Verification items for the finished model (mm, model axes). Give positions to 0.01 mm unless a question says otherwise; leave off trailing zeros. Loops run counter-clockwise (first coordinate to the right, second up) from the corner with the lowest first, then second, coordinate; pieces in that order, holes last. Notation, with made-up numbers: (14, 28) - (34, 28) arc R19 ccw to (34, 65) - close; hole circle Ø9 at (8, 21). An arc over 180 degrees is marked (long way). Answer in a Markdown table with one row per item.
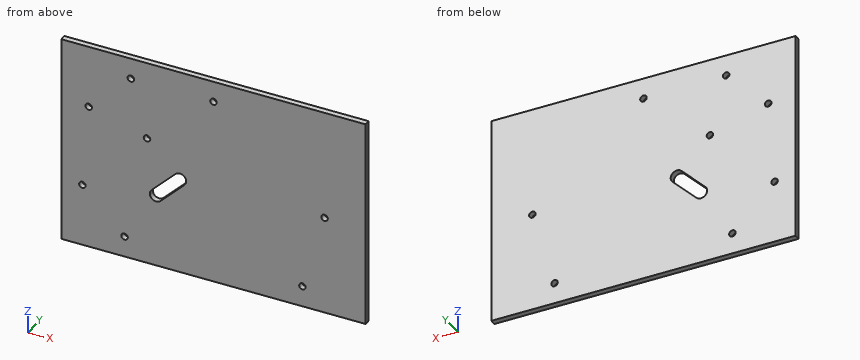
```python
from build123d import *

# Parameters (mm, degrees)
SKETCH1_W           = 144.5
SKETCH1_H           = 100
SKETCH1_R           = 1.55
BOSS_EXTRUDE1_DEPTH = 2.8
CUT_EXTRUDE1_REACH  = 4.8
CUT_EXTRUDE2_REACH  = 4.8
SKETCH3_R           = 1.55
CUT_EXTRUDE3_REACH  = 4.8
SKETCH4_R           = 1.55


with BuildPart() as part:
    # Sketch1 → Boss-Extrude1 (new body)
    with BuildSketch(Plane(origin=(0, 0, 0), x_dir=(1, 0, 0), z_dir=(0, 1, 0))):
        Rectangle(SKETCH1_W, SKETCH1_H)
        with Locations((-59.25, -20)):
            Circle(SKETCH1_R, mode=Mode.SUBTRACT)
        with Locations((-39.25, -40)):
            Circle(SKETCH1_R, mode=Mode.SUBTRACT)
        with Locations((-31.57233047, -12.32233047)):
            Circle(SKETCH1_R, mode=Mode.SUBTRACT)
    extrude(amount=BOSS_EXTRUDE1_DEPTH)

    # Sketch2 → Cut-Extrude1 (cut, up to next)
    with BuildSketch(Plane(origin=(0, 2.8, 0), x_dir=(1, 0, 0), z_dir=(0, 1, 0)), mode=Mode.PRIVATE) as cut_extrude1_sk1:
        with BuildLine():
            Line((-25.128679656, 17.121320344), (-13.814971157, 5.807611845))
            ThreePointArc((-13.814971157, 5.807611845), (-13.814971157, 1.564971157), (-18.057611845, 1.564971157))
            Line((-18.057611845, 1.564971157), (-29.371320344, 12.878679656))
            ThreePointArc((-29.371320344, 12.878679656), (-29.371320344, 17.121320344), (-25.128679656, 17.121320344))
        make_face()
    cut_extrude1_tool1 = extrude(cut_extrude1_sk1.sketch, amount=-CUT_EXTRUDE1_REACH, mode=Mode.PRIVATE) & part.part
    add(cut_extrude1_tool1.solids().sort_by_distance((-21.593146, 2.8, -9.343146))[0], mode=Mode.SUBTRACT)

    # Sketch3 → Cut-Extrude2 (cut, up to next)
    with BuildSketch(Plane(origin=(0, 2.8, 0), x_dir=(1, 0, 0), z_dir=(0, 1, 0)), mode=Mode.PRIVATE) as cut_extrude2_sk1:
        with Locations((-62.25, 20)):
            Circle(SKETCH3_R)
    cut_extrude2_tool1 = extrude(cut_extrude2_sk1.sketch, amount=-CUT_EXTRUDE2_REACH, mode=Mode.PRIVATE) & part.part
    add(cut_extrude2_tool1.solids().sort_by_distance((-62.25, 2.8, -20))[0], mode=Mode.SUBTRACT)
    # Sketch3 → Cut-Extrude2 (cut, up to next)
    with BuildSketch(Plane(origin=(0, 2.8, 0), x_dir=(1, 0, 0), z_dir=(0, 1, 0)), mode=Mode.PRIVATE) as cut_extrude2_sk2:
        with Locations((-42.25, 40)):
            Circle(SKETCH3_R)
    cut_extrude2_tool2 = extrude(cut_extrude2_sk2.sketch, amount=-CUT_EXTRUDE2_REACH, mode=Mode.PRIVATE) & part.part
    add(cut_extrude2_tool2.solids().sort_by_distance((-42.25, 2.8, -40))[0], mode=Mode.SUBTRACT)
    # Sketch3 → Cut-Extrude2 (cut, up to next)
    with BuildSketch(Plane(origin=(0, 2.8, 0), x_dir=(1, 0, 0), z_dir=(0, 1, 0)), mode=Mode.PRIVATE) as cut_extrude2_sk3:
        with Locations((42.25, 40)):
            Circle(SKETCH3_R)
    cut_extrude2_tool3 = extrude(cut_extrude2_sk3.sketch, amount=-CUT_EXTRUDE2_REACH, mode=Mode.PRIVATE) & part.part
    add(cut_extrude2_tool3.solids().sort_by_distance((42.25, 2.8, -40))[0], mode=Mode.SUBTRACT)
    # Sketch3 → Cut-Extrude2 (cut, up to next)
    with BuildSketch(Plane(origin=(0, 2.8, 0), x_dir=(1, 0, 0), z_dir=(0, 1, 0)), mode=Mode.PRIVATE) as cut_extrude2_sk4:
        with Locations((0, -40)):
            Circle(SKETCH3_R)
    cut_extrude2_tool4 = extrude(cut_extrude2_sk4.sketch, amount=-CUT_EXTRUDE2_REACH, mode=Mode.PRIVATE) & part.part
    add(cut_extrude2_tool4.solids().sort_by_distance((0, 2.8, 40))[0], mode=Mode.SUBTRACT)

    # Sketch4 → Cut-Extrude3 (cut, up to next)
    with BuildSketch(Plane(origin=(0, 2.8, 0), x_dir=(1, 0, 0), z_dir=(0, 1, 0)), mode=Mode.PRIVATE) as cut_extrude3_sk1:
        with Locations((52.75, 2.56)):
            Circle(SKETCH4_R)
    cut_extrude3_tool1 = extrude(cut_extrude3_sk1.sketch, amount=-CUT_EXTRUDE3_REACH, mode=Mode.PRIVATE) & part.part
    add(cut_extrude3_tool1.solids().sort_by_distance((52.75, 2.8, -2.56))[0], mode=Mode.SUBTRACT)


solid = part.part
```
Q1. Thickness scan on line 1 (X direction, y = 0.9, z = 40); line 2 (Z direction, x = -39.25, y = 0.85); line 3 (X direction, y = 1.45, z = -40). Record the ranges inside material, lowest first.
Completed:
| item | result |
|---|---|
| line 1 | -72.25 to -40.8, -37.7 to -1.55, 1.55 to 72.25 |
| line 2 | -50 to 38.45, 41.55 to 50 |
| line 3 | -72.25 to -43.8, -40.7 to 40.7, 43.8 to 72.25 |
Q2. Sectioned sample at B-B (z = 20). Record the cut outline in (x, y), and give its area (3 significant figures).
Completed:
| item | result |
|---|---|
| outline | (-72.25, 0) - (-60.8, 0) - (-60.8, 2.8) - (-72.25, 2.8) - close; (-57.7, 0) - (72.25, 0) - (72.25, 2.8) - (-57.7, 2.8) - close |
| area | 396 mm^2 |
Q3. Go/stop test with a flat-tipped pin: P1, Ø2.5, axis at x = 42.25, z = -40, coming from the -Y side. Record where the tip stops, or that it passes through.
Completed:
| item | result |
|---|---|
| P1 | through |
Q4. Sectioned sample at A-A (x = 52.75). Record the cut outline in (y, z).
Completed:
| item | result |
|---|---|
| outline | (0, -50) - (2.8, -50) - (2.8, -4.11) - (0, -4.11) - close; (0, -1.01) - (2.8, -1.01) - (2.8, 50) - (0, 50) - close |
